Geometry check sheet. Reference: drawing and pictorial views, mm from the part's lowest x, y, z. A direction names the side the tool comes from. Coordinates: 2 decimals unless noted, no trailing zeros. Loops run counter-clockwise (first coordinate to the right, second up) from the corner with the lowest first, then second, coordinate; pieces in that order, holes last. Notation, with made-up numbers: (34, 28) -> (49, 28) arc R12 ccw to (49, 49) -> close; hole circle Ø11 at (22.25, -2.5). An arc over 180 degrees is marked (long way). Answer as a JSON object with one key per item and string values. Group by question number.
Q1. Gauge pin test, flat ends, axial feed: pin 1 Ø1 at (y, z) = (58, 4.5) entering from +X; pin 2 Ø3 at (x, y) = (24.5, 35.5) entering from -Z; pin 3 Ø1 at (y, z) = (58, 6) entering from -X. Record the tip position at first contact, or that the pin passes through.
Q2. Cross-section at A-A on z = 9.25. Record the boundary of the cut face in (x, y), and give its area (3 significant figures).
Q3. Set-up check for the marked faces 4 and 5: record each of +Z, -Z, +X, -X, +Y, -Y from which the full face is reachable in a straight line by a thin tool's end or side.
Q4. Release check for a two-part mould opening along Y. For the marked faces 1, 2 and 3 record: released by +Y, released by -Y, zero draft, split by the parting line, or undercut.
Q5. Cross-section at C-C on y = 35. Record the boundary of the cut face in (x, z), and give its area (3 significant figures).
Q6. Cross-section at B-B on x = 23.5. Record the boundary of the cut face in (y, z).
Q7. Scan lines: L1, parallel to Y at x = 14.5, z = 2.25; L2, parallel to Z at x = 6.5, y = 7.5. Record each from-to range of solid material in increasing order.
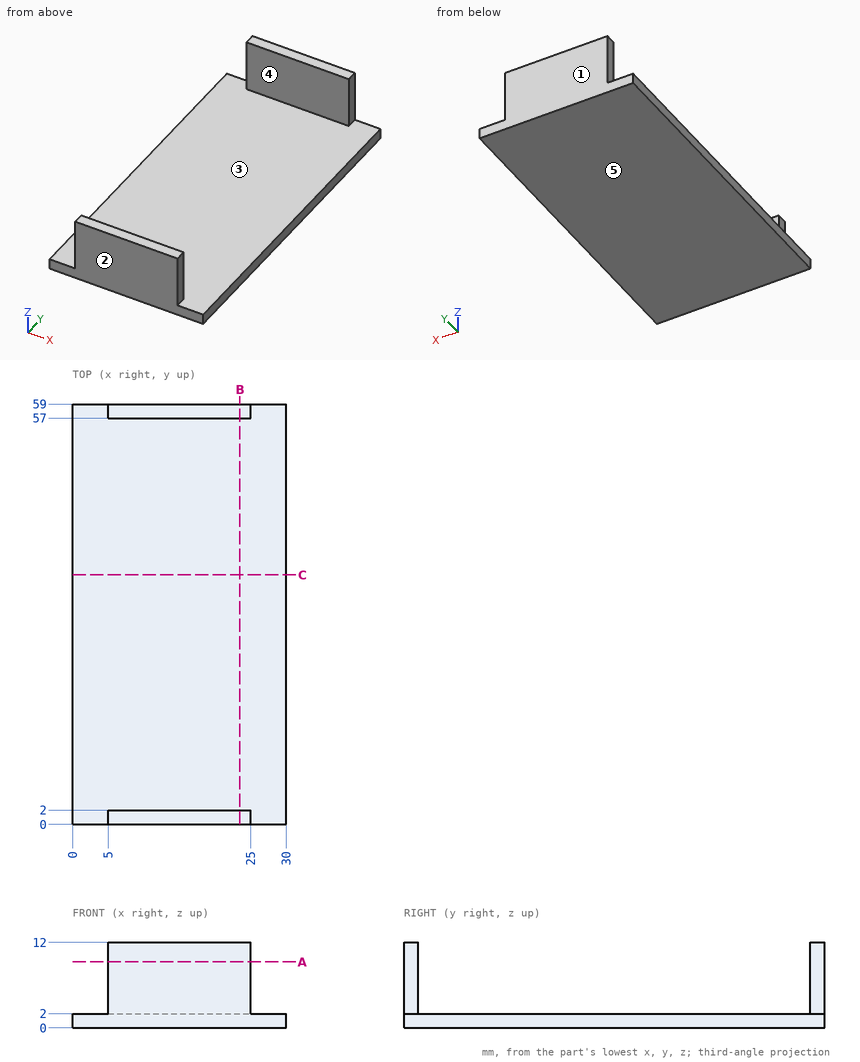
Computed values:
{
 "1": {"pin 1": "stops at x = 25", "pin 2": "stops at z = 0", "pin 3": "stops at x = 5"},
 "2": {"outline": "(5, 0) -> (25, 0) -> (25, 2) -> (5, 2) -> close; (5, 57) -> (25, 57) -> (25, 59) -> (5, 59) -> close", "area": "80.0 mm²"},
 "3": {"face 4": "+Z, +X, -X", "face 5": "-Z, +X, -X, +Y, -Y"},
 "4": {"face 1": "released by +Y", "face 2": "released by -Y", "face 3": "undercut"},
 "5": {"outline": "(0, 0) -> (30, 0) -> (30, 2) -> (0, 2) -> close", "area": "60.0 mm²"},
 "6": {"outline": "(0, 0) -> (59, 0) -> (59, 12) -> (57, 12) -> (57, 2) -> (2, 2) -> (2, 12) -> (0, 12) -> close"},
 "7": {"L1": "y = 0 to 2, 57 to 59", "L2": "z = 0 to 2"}
}
